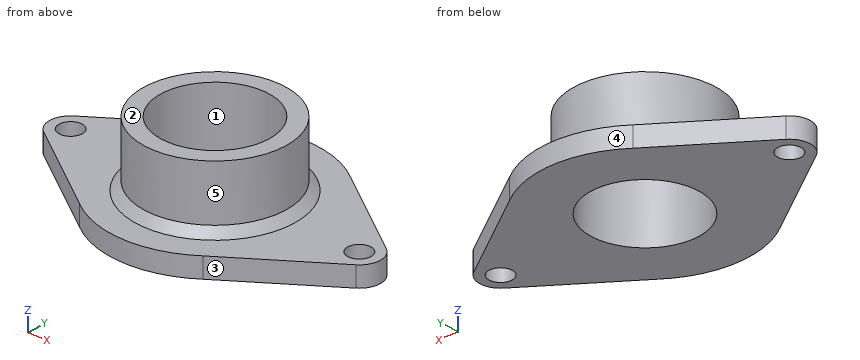
from build123d import *

# Parameters (mm, degrees)
SKETCH1_R               = 42.5
SKETCH1_R_2             = 32.5
BOSS_EXTRUDE1_DEPTH     = 50
SKETCH2_R               = 42.5
BOSS_EXTRUDE2_DEPTH     = 12
CUT_EXTRUDE1_DEPTH      = 129.086884575
CUT_EXTRUDE1_DEPTH_BACK = 129.086884575
SKETCH3_R               = 7
CHAMFER1_SIZE           = 5


with BuildPart() as part:
    # Sketch1 → Boss-Extrude1 (new body)
    with BuildSketch(Plane.XY):
        Circle(SKETCH1_R)
        Circle(SKETCH1_R_2, mode=Mode.SUBTRACT)
    extrude(amount=BOSS_EXTRUDE1_DEPTH)

    # Sketch2 → Boss-Extrude2 (add)
    with BuildSketch(Plane(origin=(0, 0, 0), x_dir=(-1, 0, 0), z_dir=(0, 0, -1))):
        with BuildLine():
            Line((-37.500000001, -49.999999999), (-94.637131817, -10.262131817))
            ThreePointArc((-94.637131817, -10.262131817), (-100, 0), (-94.637131817, 10.262131817))
            Line((-94.637131817, 10.262131817), (-37.500000001, 49.999999999))
            ThreePointArc((-37.500000001, 49.999999999), (0, 62.5), (37.500000001, 49.999999999))
            Line((37.500000001, 49.999999999), (94.637131817, 10.262131817))
            ThreePointArc((94.637131817, 10.262131817), (100, 0), (94.637131817, -10.262131817))
            Line((94.637131817, -10.262131817), (37.500000001, -49.999999999))
            ThreePointArc((37.500000001, -49.999999999), (0, -62.5), (-37.500000001, -49.999999999))
        make_face()
        Circle(SKETCH2_R, mode=Mode.SUBTRACT)
    extrude(amount=-BOSS_EXTRUDE2_DEPTH)

    # Sketch3 → Cut-Extrude1 (cut, two sides: drawn at the far end of the back side and taken through both)
    with BuildSketch(Plane(origin=(0, 0, 0), x_dir=(-1, 0, 0), z_dir=(0, 0, -1)).offset(-CUT_EXTRUDE1_DEPTH_BACK)):
        with Locations((87.5, 0)):
            Circle(SKETCH3_R)
        with Locations((-87.5, 0)):
            Circle(SKETCH3_R)
    extrude(amount=CUT_EXTRUDE1_DEPTH + CUT_EXTRUDE1_DEPTH_BACK, mode=Mode.SUBTRACT)

    # Chamfer1
    chamfer1_edges = [part.edges().sort_by_distance(p)[0] for p in [
        (-42.5, 0, 12),
    ]]
    chamfer(chamfer1_edges, length=CHAMFER1_SIZE)


solid = part.part
Can you work these out from the model? Positions are in its coordinate system, mm. Face numbers are marked on the shaded views. A direction names the side the tool comes from. Give positions to 0.01 mm unless a question says otherwise; leave off trailing zeros. Loops run counter-clockwise (first coordinate to the right, second up) from the corner with the lowest first, then second, coordinate; pieces in that order, holes last. Notation, with made-up numbers: (-7, 16.25) -> (48, 16.25) arc R14 cw to (48, 33.25) -> close; hole circle Ø1 at (74, -37.75). An arc over 180 degrees is marked (long way). Return JSON: item names as keys, results as strings.
Q1. I want a section at C-C, the plane z = 37.5. List the corners of the cut face in (x, y) for me.
Checks:
{"outline": "circle Ø85 at (0, 0); hole circle Ø65 at (0, 0)"}
Q2. For pin 1 Ø1 at (y, z) = (29.5, 20.5) entering from +X; pin 2 Ø11 at (x, y) = (-87.5, 0) entering from +Z; pin 3 Ø2 at (y, z) = (23.5, 30) entering from -X; pin 4 Ø22.5 at (x, y) = (87.5, 0) entering from +Z, each with a flat end and sliding along its axis, tell me the tip position at first contact or that it passes through.
Checks:
{"pin 1": "stops at x = 31.07", "pin 2": "passes through", "pin 3": "stops at x = -36.06", "pin 4": "stops at z = 12"}
Q3. I want a section at B-B, the plane z = 5. List the corners of the cut face in (x, y) for me, then the cut area to 3 significant figures.
Checks:
{"outline": "(-94.64, -10.26) -> (-37.5, -50) arc R62.5 ccw to (37.5, -50) -> (94.64, -10.26) arc R12.5 ccw to (94.64, 10.26) -> (37.5, 50) arc R62.5 ccw to (-37.5, 50) -> (-94.64, 10.26) arc R12.5 ccw to start; hole circle Ø14 at (-87.5, 0); hole circle Ø65 at (0, 0); hole circle Ø14 at (87.5, 0)", "area": "12,200 mm2"}
Q4. On a 3-axis mill with a long thin cutter (end or side, diameter ignored), from which of +Z, -Z, +X, -X, +Y, -Y can I reach the whole of each face in a straight line? I mean the marked faces 4 and 5. Say none if no direction works.
Checks:
{"face 4": "+Z, -Z, +Y", "face 5": "+Z"}
Q5. I want a section at D-D, the plane x = 87. List the corners of the cut face in (y, z) for me.
Checks:
{"outline": "(-15.57, 0) -> (-6.98, 0) -> (-6.98, 12) -> (-15.57, 12) -> close; (6.98, 0) -> (15.57, 0) -> (15.57, 12) -> (6.98, 12) -> close"}
Q6. I need wall thicknesses on probe 1 along Y at (x, z) = (0, 40); probe 2 along Z at (x, y) = (-79, -20); probe 3 along X at (y, z) = (24, 39). Which ranges of each line are inside material? Lowest first, please.
Checks:
{"probe 1": "y = -42.5 to -32.5, 32.5 to 42.5", "probe 2": "z = 0 to 12", "probe 3": "x = -35.07 to -21.91, 21.91 to 35.07"}
Q7. We'd pull the mould along Y, two halves only. Please class the marked faces 1, 2 and 3: released by +Y, released by -Y, zero draft, split by the parting line, or undercut.
Checks:
{"face 1": "undercut", "face 2": "zero draft", "face 3": "released by -Y"}
Q8. I want a section at A-A, the plane x = 0. List the corners of the cut face in (y, z) for me, then the cut area to 4 significant figures.
Checks:
{"outline": "(-62.5, 0) -> (-32.5, 0) -> (-32.5, 50) -> (-42.5, 50) -> (-42.5, 17) -> (-47.5, 12) -> (-62.5, 12) -> close; (32.5, 0) -> (62.5, 0) -> (62.5, 12) -> (47.5, 12) -> (42.5, 17) -> (42.5, 50) -> (32.5, 50) -> close", "area": "1,505 mm2"}
